from build123d import *

# Parameters (mm, degrees)
F0_W     = 63.5
F0_H     = 88.9
F0_R     = 3.937
F0_R_2   = 7.4295
F1_DEPTH = 19.05
F2_R     = 11.3792
F2_R_2   = 7.4295
F3_DEPTH = 2.54


with BuildPart() as f1:
    # F0 (on Top) → F1 (new body)
    with BuildSketch(Plane.XY):
        with Locations((31.75, 44.45)):
            Rectangle(F0_W, F0_H)
        with Locations((31.75, 11.176)):
            Circle(F0_R, mode=Mode.SUBTRACT)
        with Locations((13.5382, 59.944)):
            Circle(F0_R_2, mode=Mode.SUBTRACT)
        with Locations((11.43, 81.28)):
            Circle(F0_R, mode=Mode.SUBTRACT)
        with Locations((49.9618, 59.944)):
            Circle(F0_R_2, mode=Mode.SUBTRACT)
        with Locations((52.07, 81.28)):
            Circle(F0_R, mode=Mode.SUBTRACT)
    extrude(amount=F1_DEPTH)

    # F2 (on face) → F3 (cut)
    with BuildSketch(Plane(origin=(0, 0, 0), x_dir=(1, 0, 0), z_dir=(0, 0, -1))):
        with Locations((49.9618, -59.944)):
            Circle(F2_R)
        with Locations((49.9618, -59.944)):
            Circle(F2_R_2, mode=Mode.SUBTRACT)
        with Locations((13.5382, -59.944)):
            Circle(F2_R)
        with Locations((13.5382, -59.944)):
            Circle(F2_R_2, mode=Mode.SUBTRACT)
    extrude(amount=-F3_DEPTH, mode=Mode.SUBTRACT)


with BuildPart() as f4_1:
    # F4: copy of F1
    add(f1.part.moved(Location((-152.4, 0, 0))))


solid = f1.part
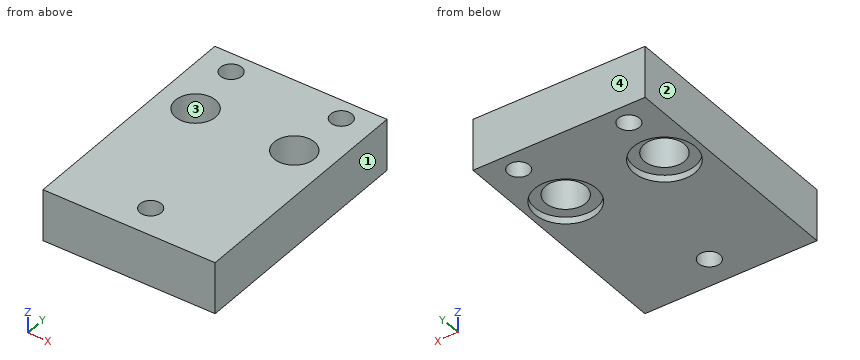
Read the model definition and answer for the solid it produces. Units are mm, in the model's axes. Face numbers are marked on the shaded views. Give positions to 0.01 mm unless a question says otherwise; leave off trailing zeros. Write each loop counter-clockwise with the first axis right and the second up, starting at its lowest first coordinate (ties: lowest second). Pieces come first, ordered by that corner, then holes. Notation, with made-up numbers: (84.5, -0.5) - (131.5, -0.5) arc R9 ccw to (131.5, 4.5) - close; hole circle Ø1 at (-20.5, 68). An arc over 180 degrees is marked (long way). Use CSV: the item, a comma, the result in double quotes. Start each with the question number.
Item 1: The part is cut by section D-D, the plane z = 17.5. Give the vertices of the cut face in (x, y).
Item 2: The part is cut by section B-B, the plane x = 31.75. Give the vertices of the cut face in (y, z), and give its area (3 significant figures).
Item 3: A flat-ended cylindrical pin translates along its axis: P1, Ø7, axis at x = 13.5, y = 55.5, coming from the -Z side. Find the tip coordinate at first contact, or state that the pin passes through.
Item 4: Consider line 1 (Y direction, x = 11.43, z = 6); line 2 (X direction, y = 65, z = 1.5); line 3 (Y direction, x = 29, z = 8.75). Determine where each line is inside the solid, lowest interval first.
Item 5: The part is cut by section A-A, the plane y = 81.28. Give the vertices of the cut face in (x, z), and give its area (3 significant figures).
Item 6: The part is cut by section C-C, the plane x = 51. Give the vertices of the cut face in (y, z).
Item 7: The mould has two halves that part along X. Classify the marked faces 1, 2, 3 and 4: pulls with the +X half, pulls with the -X half, needs draft (parallel to the pull), parting line crosses it, or undercut.
Taken from the geometry:
1,outline,"(0, 0) - (63.5, 0) - (63.5, 88.9) - (0, 88.9) - close; hole circle Ø14.86 at (13.54, 59.94); hole circle Ø7.87 at (11.43, 81.28); hole circle Ø7.87 at (31.75, 11.18); hole circle Ø14.86 at (49.96, 59.94); hole circle Ø7.87 at (52.07, 81.28)"
2,outline,"(0, 0) - (7.24, 0) - (7.24, 19.05) - (0, 19.05) - close; (15.11, 0) - (88.9, 0) - (88.9, 19.05) - (15.11, 19.05) - close"
2,area,"1,540 mm2"
3,P1,"z = 2.54"
4,line 1,"0 to 52.82, 67.07 to 77.34, 85.22 to 88.9"
4,line 2,"0 to 3.34, 23.73 to 39.77, 60.16 to 63.5"
4,line 3,"0 to 8.36, 13.99 to 88.9"
5,outline,"(0, 0) - (7.49, 0) - (7.49, 19.05) - (0, 19.05) - close; (15.37, 0) - (48.13, 0) - (48.13, 19.05) - (15.37, 19.05) - close; (56.01, 0) - (63.5, 0) - (63.5, 19.05) - (56.01, 19.05) - close"
5,area,"910 mm2"
6,outline,"(0, 0) - (48.61, 0) - (48.61, 2.54) - (52.59, 2.54) - (52.59, 19.05) - (0, 19.05) - close; (67.3, 2.54) - (71.28, 2.54) - (71.28, 0) - (77.49, 0) - (77.49, 19.05) - (67.3, 19.05) - close; (85.07, 0) - (88.9, 0) - (88.9, 19.05) - (85.07, 19.05) - close"
7,face 1,"pulls with the +X half"
7,face 2,"pulls with the -X half"
7,face 3,"undercut"
7,face 4,"needs draft"
